The listing builds one solid part. Answer for the finished solid, in the listing's coordinates (mm). A direction names the side the tool comes from. Give positions to 0.01 mm unless a question says otherwise; leave off trailing zeros. Write each loop counter-clockwise with the first axis right and the second up, starting at its lowest first coordinate (ties: lowest second). Pieces come first, ordered by that corner, then holes. Notation, with made-up numbers: M 73,86.5 L 125,86.5 A23 ccw 125,101.5 Z; hole C 3,9 d2. An arc over 180 degrees is marked long. Return JSON: item names as keys, results as strings.
from build123d import *

# Parameters (mm, degrees)
SKETCH1_R           = 8
BOSS_EXTRUDE1_DEPTH = 66
BOSS_EXTRUDE2_DEPTH = 22.5


with BuildPart() as part:
    # Sketch1 → Boss-Extrude1 (new body)
    with BuildSketch(Plane.XY):
        Circle(SKETCH1_R)
    extrude(amount=BOSS_EXTRUDE1_DEPTH)

    # Sketch2 → Boss-Extrude2 (add, symmetric)
    with BuildSketch(Plane.XY.offset(33)):
        with BuildLine():
            Line((-10.662181086, 42.002247261), (-19.468214294, 4.581335198))
            ThreePointArc((-19.468214294, 4.581335198), (0, -20), (19.468214294, 4.581335198))
            Line((19.468214294, 4.581335198), (10.662181086, 42.002247261))
            ThreePointArc((10.662181086, 42.002247261), (0, 50.44660655), (-10.662181086, 42.002247261))
        make_face()
    extrude(amount=BOSS_EXTRUDE2_DEPTH, both=True)


solid = part.part
Item 1: A cutting plane is placed at A-A, the plane x = 0. Write down the section's boundary in (y, z), plus the area to 3 significant figures.
Geometry results:
{"outline": "M -20,10.5 L -8,10.5 L -8,0 L 8,0 L 8,10.5 L 50.45,10.5 L 50.45,55.5 L 8,55.5 L 8,66 L -8,66 L -8,55.5 L -20,55.5 Z", "area": "3,510 mm2"}
Item 2: Find the intervals of material crossed by line 1 (Z direction, x = -4, y = -13.5); line 2 (Y direction, x = 0, z = 18); line 3 (X direction, y = 37.5, z = 44), in increasing order.
Geometry results:
{"line 1": "z = 10.5 to 55.5", "line 2": "y = -20 to 50.45", "line 3": "x = -11.72 to 11.72"}
Item 3: Given pin 1 Ø12 at (x, y) = (13, -1.5) entering from -Z; pin 2 Ø5 at (x, z) = (-8.5, 16) entering from -Y; pin 3 Ø4 at (y, z) = (11, 12.5) entering from -X; pin 4 Ø5 at (x, y) = (14, 28.5) entering from +Z, each flat-ended and moving along its own axis, determine where each tip first touches the part or whether it passes through.
Geometry results:
{"pin 1": "stops at z = 0", "pin 2": "stops at y = -19.08", "pin 3": "stops at x = -18.43", "pin 4": "stops at z = 55.5"}
Item 4: A cutting plane is placed at D-D, the plane y = 26. Write down the section's boundary in (x, z).
Geometry results:
{"outline": "M -14.43,10.5 L 14.43,10.5 L 14.43,55.5 L -14.43,55.5 Z"}
Item 5: A cutting plane is placed at C-C, the plane z = 43. Write down the section's boundary in (x, y).
Geometry results:
{"outline": "M -19.47,4.58 A20 ccw long 19.47,4.58 L 10.66,42 A10.95 ccw -10.66,42 Z"}
Item 6: Which of the six approach directions +Z, -Z, +X, -X, +Y, -Y give full straight-line access (tool end or side, diameter ignored) to faces 1 (the cylindrical face through (-1.73, -7.81, 5.18)), 2 (the flat face through (-15.004, 23.554, 33.315)), 3 (the cylindrical face through (-1.73, -7.81, 60.68))?
Geometry results:
{"face 1": "-Z", "face 2": "+Z, -Z, -X, +Y", "face 3": "+Z"}
Item 7: A cutting plane is placed at B-B, the plane y = 0. Write down the section's boundary in (x, z).
Geometry results:
{"outline": "M -20,10.5 L -8,10.5 L -8,0 L 8,0 L 8,10.5 L 20,10.5 L 20,55.5 L 8,55.5 L 8,66 L -8,66 L -8,55.5 L -20,55.5 Z"}
